Check sheet for the modelled part. Datum: model origin and axes. Units: mm. Coordinates: 2 decimals unless noted, no trailing zeros. Loops run counter-clockwise (first coordinate to the right, second up) from the corner with the lowest first, then second, coordinate; pieces in that order, holes last. Notation, with made-up numbers: (82.5, -15.75) -> (87.5, -15.75) arc R19 ccw to (87.5, -9.75) -> close; hole circle Ø4 at (78.25, -28). An arc over 180 degrees is marked (long way). Use CSV: the item, a comma, the result in double quotes.
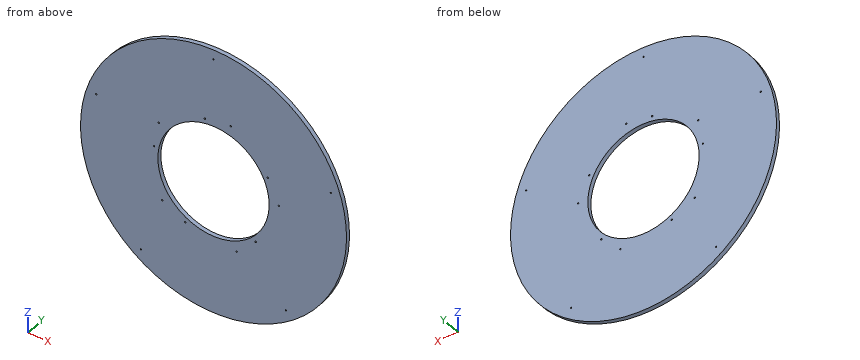
Autodesk Inventor part; units mm, degrees
ref_plane "YZ Plane" through (0, 0, 0) normal (1, 0, 0) x (0, 1, 0)
ref_plane "XZ Plane" through (0, 0, 0) normal (0, 1, 0) x (-1, 0, 0)
ref_plane "XY Plane" through (0, 0, 0) normal (0, 0, 1) x (1, 0, 0)
sketch "Sketch1" plane through (0, 0, 0) normal (0, 1, 0) x (-1, 0, 0)
  line L0 (1200, -600) -> (-1200, -600)
  line L1 (-1200, -600) -> (-1200, 600)
  line L2 (-1200, 600) -> (1200, 600)
  line L3 (1200, 600) -> (1200, -600)
  line L4 (1200, -600) -> (-1200, 600) construction
  line L5 (-1200, -600) -> (1200, 600) construction
  circle A0 centre (0, 0) radius 130 construction
  circle A1 centre (0, 0) radius 325 construction
  line L6 (0, 325) -> (309.0934, 100.4305) construction
  line L7 (309.0934, 100.4305) -> (191.0302, -262.9305) construction
  line L8 (191.0302, -262.9305) -> (-191.0302, -262.9305) construction
  line L9 (-191.0302, -262.9305) -> (-309.0934, 100.4305) construction
  line L10 (-309.0934, 100.4305) -> (0, 325) construction
  line L11 (0, 0) -> (0, 325) construction
  line L12 (0, 0) -> (-309.0934, 100.4305) construction
  line L13 (0, 0) -> (-191.0302, -262.9305) construction
  line L14 (0, 0) -> (309.0934, 100.4305) construction
  line L15 (0, 0) -> (191.0302, -262.9305) construction
  arc A2 (-15.7737, 293.9464) -> (0, 0) centre (281.4583, 162.5) ccw
  arc A3 (224.7845, 110.9324) -> (0, 0) centre (230.7976, -184.461) ccw
  arc A4 (275.3692, 201.188) -> (35.5667, 329.5753) centre (50.8772, 70.0265) ccw
  arc A5 (224.7845, 110.9324) -> (275.3692, 201.188) centre (223.5633, 170.92) ccw
  arc A6 (35.5667, 329.5753) -> (-15.7737, 293.9464) centre (39.0999, 269.6794) ccw
  arc A7 (-284.434, 75.8328) -> (0, 0) centre (-67.5713, 317.898) ccw
  arc A8 (-36.0407, 248.0627) -> (0, 0) centre (246.7532, 162.5) ccw
  arc A9 (-106.2474, 324.0622) -> (-302.454, 135.6703) centre (-50.8772, 70.0265) ccw
  arc A10 (-36.0407, 248.0627) -> (-106.2474, 324.0622) centre (-93.4697, 265.4385) ccw
  arc A11 (-302.454, 135.6703) -> (-284.434, 75.8328) centre (-244.3978, 120.5217) ccw
  arc A12 (-160.0162, -247.0792) -> (0, 0) centre (-323.2196, 33.9718) ccw
  arc A13 (-247.0589, 42.3788) -> (0, 0) centre (-78.2958, 284.8915) ccw
  arc A14 (-341.0337, -0.9066) -> (-222.4935, -245.7264) centre (-82.321, -26.7477) ccw
  arc A15 (-247.0589, 42.3788) -> (-341.0337, -0.9066) centre (-281.3308, -6.8699) ccw
  arc A16 (-222.4935, -245.7264) -> (-160.0162, -247.0792) centre (-190.146, -195.1929) ccw
  arc A17 (185.5386, -228.5361) -> (0, 0) centre (-132.1894, -296.9023) ccw
  arc A18 (-116.65, -221.8712) -> (0, 0) centre (-295.1426, 13.5726) ccw
  arc A19 (-104.523, -324.6224) -> (164.9454, -287.5376) centre (0, -86.5575) ccw
  arc A20 (-116.65, -221.8712) -> (-104.523, -324.6224) centre (-80.4023, -269.6844) ccw
  arc A21 (164.9454, -287.5376) -> (185.5386, -228.5361) centre (126.8811, -241.1575) ccw
  arc A22 (274.6853, 105.8361) -> (0, 0) centre (241.5221, -217.4674) ccw
  arc A23 (174.9652, -179.5027) -> (0, 0) centre (-104.1124, -276.5031) ccw
  arc A24 (276.4349, -199.7211) -> (324.4354, 68.0184) centre (82.321, -26.7477) ccw
  arc A25 (174.9652, -179.5027) -> (276.4349, -199.7211) centre (231.6394, -159.8042) ccw
  arc A26 (324.4354, 68.0184) -> (274.6853, 105.8361) centre (268.5629, 46.1493) ccw
  line L16 (246.7532, 162.5) -> (-78.2958, 284.8915)
  line L17 (-78.2958, 284.8915) -> (-295.1426, 13.5726)
  line L18 (-295.1426, 13.5726) -> (-104.1124, -276.5031)
  line L19 (-104.1124, -276.5031) -> (230.7976, -184.461)
  line L20 (230.7976, -184.461) -> (246.7532, 162.5)
  circle A27 centre (0, 0) radius 251.1364
  circle A28 centre (223.5633, 170.92) radius 60 construction
  circle A29 centre (246.7532, 162.5) radius 43.2425 construction
  circle A30 centre (246.7532, 162.5) radius 3.18
  circle A31 centre (39.0999, 269.6794) radius 3.5
  circle A32 centre (-78.2958, 284.8915) radius 3.18
  circle A33 centre (-244.3978, 120.5217) radius 3.5
  circle A34 centre (-295.1426, 13.5726) radius 3.18
  circle A35 centre (-190.146, -195.1929) radius 3.5
  circle A36 centre (-104.1124, -276.5031) radius 3.18
  circle A37 centre (126.8811, -241.1575) radius 3.5
  circle A38 centre (230.7976, -184.461) radius 3.18
  circle A39 centre (268.5629, 46.1493) radius 3.18
  point P0 (-309.0934, 100.4305)
  point P1 (0, 325)
  point P2 (-191.0302, -262.9305)
  point P3 (-309.0934, 100.4305)
  point P4 (191.0302, -262.9305)
  point P5 (-191.0302, -262.9305)
  point P6 (309.0934, 100.4305)
  point P7 (191.0302, -262.9305)
  dimension "d3" = 650
  dimension "d0" = 2400
  dimension "d1" = 1200
  dimension "d2" = 260
  dimension "d9" = 325
  dimension "d10" = 295.4545
  dimension "d11" = 260
  dimension "d12" = 60
  dimension "d15" = 360
  dimension "d21" = 502.2727
  dimension "d22" = 6.36
  dimension "d23" = 7
  dimension "d24" = 6.36
  dimension "d25" = 7
  dimension "d26" = 6.36
  dimension "d27" = 7
  dimension "d28" = 6.36
  dimension "d29" = 7
  dimension "d30" = 6.36
  dimension "d31" = 6.36
extrude "Extrusion1" add sketch "Sketch1" along normal blind 19 contours L0 L1 L2 L3 | A6 A4 A5 L20 A30 L16 A27 A2 | L16 A27 A2 | A2 A27 A10 L16 | A27 L16 A5 A3 A2 | A2 A8 A10 A27 | A27 L16 | L16 A32 L17 A27 A7 A11 A9 A10 | A10 A27 L17 A32 L16 | A13 A15 A27 A7 | A7 A27 L17 A10 A8 | A18 A20 A27 A12 | A12 A27 L18 A15 A13 | A23 A25 A27 A17 | A17 A27 L19 A20 A18 | A3 A5 A27 A22 | A22 A27 L20 A25 A23 | L16 A30 L20 A5 A27 | A32 L17 L16 | L16 L17 A32 | L20 A22 A27 A5 | A27 A15 L17 A7 | A7 L17 A27 | A27 A20 L18 A12 | A12 L18 A27 | A27 A25 L19 A17 | A17 L19 A27 | A22 L20 A27 | L17 A27 | A30 L20 L16 | L16 L20 A30 | A22 A26 A24 A25 L19 A38 L20 A27 | A27 L18 A34 L17 A15 | A12 A16 A14 A15 L17 A34 L18 A27 | A27 L18 | A27 L19 A36 L18 A20 | A17 A21 A19 A20 L18 A36 L19 A27 | A27 L19 | A27 L20 A38 L19 A25 | A27 L20 | A34 L18 L17 | L17 L18 A34 | A36 L19 L18 | L18 L19 A36 | A38 L20 L19 | L19 L20 A38 | A31 | A33 | A35 | A37 | A39
extrude "Extrusion3" cut sketch "Sketch1" along normal blind 19 contours A32 L17 L16 | L16 L17 A32 | A30 L20 L16 | L16 L20 A30 | A34 L18 L17 | L17 L18 A34 | A36 L19 L18 | L18 L19 A36 | A38 L20 L19 | L19 L20 A38 | A31 | A33 | A35 | A37 | A39
sketch "Sketch3" plane through (0, 0, 0) normal (0, -1, 0) x (1, 0, 0)
  circle A0 centre (0, 0) radius 251.1364
extrude "Extrusion4" cut sketch "Sketch3" against normal up to next
sketch "Sketch7" plane through (0, 0, 0) normal (0, -1, 0) x (1, 0, 0)
  arc A0 (-0.1434, 553) -> (-0.1452, 560) centre (-0.1443, 556.5) ccw
  circle A1 centre (-0.1443, 556.5) radius 3.18
  dimension "d50" = 6.36
extrude "Extrusion8" cut sketch "Sketch7" against normal blind 19
pattern_circular "Circular Pattern1" count 5 over 360 about axis through (0, 0, 0) along (0, 1, 0) of "Extrusion8"
sketch "Sketch8" plane through (0, 0, 0) normal (0, -1, 0) x (1, 0, 0)
  circle A0 centre (0, 0) radius 251.1364
  line L0 (-1200, -600) -> (1200, -600)
  line L1 (1200, -600) -> (1200, 600)
  line L2 (1200, 600) -> (-1200, 600)
  line L3 (-1200, 600) -> (-1200, -600)
  circle A1 centre (0, 0) radius 600
  dimension "d47" = 1200
extrude "Extrusion9" cut sketch "Sketch8" against normal blind 19 contours A0 | L3 L2 A1 L0 | A1 L2 L1 L0
equation "\"d2\" = 0.4 * d3"
equation "\"d9\" = 0.5 * d3"
equation "\"d10\" = 0.454545 * d3"
equation "\"d11\" = 0.4 * d3"
equation "\"d21\" = 1.7 * d10"
equation "\"d24\" = d22"
equation "\"d26\" = d28"
equation "\"d28\" = d30"
equation "\"d30\" = d31"
equation "\"d31\" = d22"
properties part number "plancha"
1) Cross-section at B-B on y = 3.75. Give the number of separate pieces and of enclosed holes in the cut face, and give its area (3 significant figures).
Answer below:
separate pieces,"1"
enclosed holes,"16"
area,"932,000 mm²"
2) Cross-section at D-D on z = 346.5. Record the boundary of the cut face in (x, y).
Answer below:
outline,"(-489.83, 0) -> (489.83, 0) -> (489.83, 19) -> (-489.83, 19) -> close"
3) Go/stop test with flat-tipped pins: pin 1 Ø5.5 at (x, z) = (104.11, -276.5) entering from -Y; pin 2 Ø1.5 at (y, z) = (2, -42.5) entering from +X; pin 3 Ø8 at (x, y) = (349.5, 13.5) entering from -Z; pin 4 Ø6 at (y, z) = (16.5, 83.5) entering from +X. Record where each tip stops, or that it passes through.
Answer below:
pin 1,"passes through"
pin 2,"stops at x = 598.55"
pin 3,"stops at z = -490.54"
pin 4,"stops at x = 594.58"
4) Cross-section at C-C on z = 95. Record the boundary of the cut face in (x, y).
Answer below:
outline,"(-592.43, 0) -> (-232.47, 0) -> (-232.47, 19) -> (-592.43, 19) -> close; (232.47, 0) -> (592.43, 0) -> (592.43, 19) -> (232.47, 19) -> close"
5) Cross-section at A-A on x = -109. Record the boundary of the cut face in (y, z).
Answer below:
outline,"(0, -590.02) -> (19, -590.02) -> (19, -226.25) -> (0, -226.25) -> close; (0, 226.25) -> (19, 226.25) -> (19, 590.02) -> (0, 590.02) -> close"
6) Thickness scan on line 1 along X through (y, z) = (17.75, -12); line 2 along Z through (x, y) = (-180, 6.25); line 3 along Z through (x, y) = (327, 12.5). Record the ranges inside material, lowest first. Write a range as from..to.
Answer below:
line 1,"x = -599.88..-250.85, 250.85..599.88"
line 2,"z = -572.36..-175.13, 175.13..572.36"
line 3,"z = -503.06..-453.31, -446.96..503.06"
